Read the model definition and answer for the solid it produces. Units are mm, in the model's axes. A direction names the side the tool comes from. Coordinates: 2 decimals unless noted, no trailing zeros. Write each loop counter-clockwise with the first axis right and the second up, starting at its lowest first coordinate (ties: lowest second). Pieces come first, ordered by that corner, then holes. Notation, with made-up numbers: (1.5, -29) -> (46.5, -29) arc R23 ccw to (46.5, -17) -> close; hole circle Ø3 at (-24.5, 39.5). An arc over 180 degrees is marked (long way). Use CSV: the item, a comma, the result in double quotes.
from build123d import *

# Parameters (mm, degrees)
EXTRUDE_1_DEPTH        = 6
HOLE_WIZARD_M6_1_D     = 5
HOLE_WIZARD_M6_1_DEPTH = 18
HOLE_WIZARD_M6_1_TIP   = 1.502151548
SKETCH_4_R             = 9
CUT_EXTRUDE_1_DEPTH    = 13
FILLET_1_R             = 10


with BuildPart() as part:
    # 草图1 → 凸台-拉伸1 (new body, symmetric)
    with BuildSketch(Plane.XY):
        Polygon((0, 0), (75, 0), (75, 12), (120, 12), (120, 44), (0, 44), align=None)
    extrude(amount=EXTRUDE_1_DEPTH, both=True)

    # M6 螺纹孔1
    with Locations(Plane(origin=(0, 0, 0), x_dir=(-1, 0, 0), z_dir=(0, -1, 0))):
        with Locations((-10, 0), (-65, 0)):
            Hole(HOLE_WIZARD_M6_1_D / 2, depth=HOLE_WIZARD_M6_1_DEPTH)
            with Locations((0, 0, -(HOLE_WIZARD_M6_1_DEPTH + HOLE_WIZARD_M6_1_TIP / 2))):  # 118° drill point
                Cone(0, HOLE_WIZARD_M6_1_D / 2, HOLE_WIZARD_M6_1_TIP, mode=Mode.SUBTRACT)

    # 草图4 → 切除-拉伸1 (cut, through all)
    with BuildSketch(Plane.XY.offset(6)):
        with Locations((105, 28)):
            Circle(SKETCH_4_R)
    extrude(amount=-CUT_EXTRUDE_1_DEPTH, mode=Mode.SUBTRACT)

    # 圆角1
    fillet_1_edges = [part.edges().sort_by_distance(p)[0] for p in [
        (0, 44, 0),
        (120, 44, 0),
        (120, 12, 0),
        (75, 12, 0),
    ]]
    fillet(fillet_1_edges, radius=FILLET_1_R)


solid = part.part
1. A cutting plane is placed at C-C (y = 16.5). Give the vertices of the cut face in (x, z), and give its area (3 significant figures).
Solutions:
outline,"(0, -6) -> (118.35, -6) -> (118.35, 6) -> (0, 6) -> close; hole circle Ø5 at (10, 0); hole circle Ø5 at (65, 0)"
area,"1,380 mm^2"
2. Each of these flat-tipped pins is pushed along its axis until it touches: pin 1 Ø1.6 at (y, z) = (0.5, 0) entering from +X; pin 2 Ø1 at (y, z) = (6.5, -1.5) entering from +X; pin 3 Ø4 at (x, z) = (10, 0) entering from -Y. Where does it stop, or does it pass through?
Solutions:
pin 1,"stops at x = 75"
pin 2,"stops at x = 76.34"
pin 3,"stops at y = 18.3"
3. Find the intervals of material crossed by line 1 along X through (y, z) = (4, 0.75); line 2 along Z through (x, y) = (65, 3); line 3 along X through (y, z) = (17.5, 1), in increasing order.
Solutions:
line 1,"x = 0 to 7.62, 12.38 to 62.62, 67.38 to 75.2"
line 2,"z = -6 to -2.5, 2.5 to 6"
line 3,"x = 0 to 7.71, 12.29 to 62.71, 67.29 to 118.93"
4. For a pull along X with two mould halves and no side action, classify faces 4 (the cylindrical face through (2.85, 40.99, -0.08)), 5 (the cylindrical face through (67.385, 9.126, -0.751)), 6 (the cylindrical face through (77.85, 8.99, 0.08)) as pulls with the +X half, pulls with the -X half, needs draft (parallel to the pull), parting line crosses it, or undercut.
Solutions:
face 4,"pulls with the -X half"
face 5,"undercut"
face 6,"pulls with the +X half"
5. A cutting plane is placed at D-D (y = 6). Give the vertices of the cut face in (x, z), and give its area (3 significant figures).
Solutions:
outline,"(0, -6) -> (75.83, -6) -> (75.83, 6) -> (0, 6) -> close; hole circle Ø5 at (10, 0); hole circle Ø5 at (65, 0)"
area,"871 mm^2"
6. A cutting plane is placed at B-B (x = 105). Give the vertices of the cut face in (y, z).
Solutions:
outline,"(12, -6) -> (19, -6) -> (19, 6) -> (12, 6) -> close; (37, -6) -> (44, -6) -> (44, 6) -> (37, 6) -> close"
7. A cutting plane is placed at A-A (y = 28). Give the vertices of the cut face in (x, z), and give its area (3 significant figures).
Solutions:
outline,"(0, -6) -> (96, -6) -> (96, 6) -> (0, 6) -> close; (114, -6) -> (120, -6) -> (120, 6) -> (114, 6) -> close"
area,"1,220 mm^2"
8. A tool of negligible diameter and unlimited length cuts with its end or side. For faces 1 (the flat face through (59, 22, 6)), 2 (the flat face through (97, 12, 0)), 3 (the cylindrical face through (7.5, 9.1, -0.1)), from which of +Z, -Z, +X, -X, +Y, -Y can it reach the whole face along a straight path? Write none if from no direction.
Solutions:
face 1,"+Z, +X, -X, +Y, -Y"
face 2,"+Z, -Z, +X, -Y"
face 3,"-Y"
